```python
from build123d import *

# Parameters (mm, degrees)
EXTRUDE_1_DEPTH      = 3.7
EXTRUDE_1_DEPTH_BACK = 3.7
SKETCH_3_R           = 2.5
CUT_EXTRUDE_1_DEPTH  = 5
SKETCH_4_R           = 1.25
EXTRUDE_2_DEPTH      = 7
FILLET_1_R           = 1
FILLET_2_R           = 0.2


with BuildPart() as part:
    # 草图2 → 凸台-拉伸1 (new, two sides: drawn at the far end of the back side and taken through both)
    with BuildSketch(Plane(origin=(0, 0, 0), x_dir=(1, 0, 0), z_dir=(0, 1, 0)).offset(-EXTRUDE_1_DEPTH_BACK)):
        Polygon((12, 4.5), (12, -4.5), (0, -4.5), (-9, -4), (-13, -4), (-13, 4), (-9, 4), (0, 4.5), align=None)
    extrude(amount=EXTRUDE_1_DEPTH + EXTRUDE_1_DEPTH_BACK)

    # 草图3 → 切除-拉伸1 (cut)
    with BuildSketch(Plane(origin=(12, 0, 0), x_dir=(0, 0, -1), z_dir=(1, 0, 0))):
        Circle(SKETCH_3_R)
    extrude(amount=-CUT_EXTRUDE_1_DEPTH, mode=Mode.SUBTRACT)

    # 草图4 → 凸台-拉伸2 (add)
    with BuildSketch(Plane(origin=(7, 0, 0), x_dir=(0, 0, -1), z_dir=(1, 0, 0))):
        with Locations(Location((0, 0, 0), (0, 0, 180))):
            Circle(SKETCH_4_R)
    extrude(amount=EXTRUDE_2_DEPTH)

    # 圆角1
    fillet_1_edges = [part.edges().sort_by_distance(p)[0] for p in [
        (12, 0, -4.5),
        (12, 0, 4.5),
    ]]
    fillet(fillet_1_edges, radius=FILLET_1_R)

    # 圆角2
    fillet_2_edges = [part.edges().sort_by_distance(p)[0] for p in [
        (14, 0, -1.25),
    ]]
    fillet(fillet_2_edges, radius=FILLET_2_R)

    # 草图5 → 旋转1 (revolve)
    with BuildSketch(Plane(origin=(0, 0, 0), x_dir=(1, 0, 0), z_dir=(0, 1, 0))):
        Polygon((-13, 2.9), (-43, 2), (-43, 0), (-13, 0), align=None)
    revolve(axis=Axis((5.484305881, 0, 0), (-1, 0, 0)))


solid = part.part
```
For this review, take the finished solid that the model builds, in its own axes (mm). A direction names the side the tool comes from. Coordinates: 2 decimals unless noted, no trailing zeros. Write each loop counter-clockwise with the first axis right and the second up, starting at its lowest first coordinate (ties: lowest second). Pieces come first, ordered by that corner, then holes. Notation, with made-up numbers: (-31.75, 77.5) - (15.25, 77.5) arc R35 cw to (15.25, 111.5) - close; hole circle Ø6 at (67, -22.75). An arc over 180 degrees is marked (long way). Answer in a Markdown table with one row per item. Add a question column.
Q1. We need section A-A, the plane y = 0. State the section outline as (x, z) points.
Q2. Tool access review of faces 1 (the conical face through (-28.21, 2.386, 0.53)), 2 (the flat face through (7, -1, 1)), 3 (the flat face through (-11, 0, -4)), 4 (the flat face through (-11, 0, 4)): name each direction out of +Z, -Z, +X, -X, +Y, -Y from which nothing blocks a thin tool from reaching the whole face with its end or side.
Q3. For P1, Ø1.5, axis at y = -0.5, z = -1, coming from the +X side; P2, Ø2, axis at x = -11.5, y = 1, coming from the +Z side; P3, Ø1.2, axis at x = -11, y = 0.5, coming from the -Z side, all flat-tipped, find the tip position at first contact; note any pin that passes through.
Q4. We need section D-D, the plane x = -19.5. State the section outline as (y, z) points (3 decimals).
Q5. For probe 1 along Y at (x, z) = (9.4, 0); probe 2 along X at (y, z) = (3, 2); probe 3 along Z at (x, y) = (8, 2), list the stretches that pass through material, from the lowest coordinate up.
Q6. We need section B-B, the plane z = 0. State the section outline as (x, y) points, and give its area (3 significant figures).
Q7. We need section C-C, the plane x = -38. State the section outline as (y, z) points, and give its area (3 significant figures).
Q8. Draft analysis for pull direction Z (two halves, no side actions). For faces 5 (the cylindrical face through (10.35, -0.05, -1.25)), 6 (the flat face through (-4.563, -0.052, -4.246)), 7 (the flat face through (12, -3, 0)), state which applies: +Z half, -Z half, draft (parallel to the pull), parting line (faces both ways), or undercut.
Answer list:
| question | item | result |
|---|---|---|
| 1 | outline | (-43, -2) - (-13, -2.9) - (-13, -4) - (-9, -4) - (0, -4.5) - (11, -4.5) arc R1 ccw to (12, -3.5) - (12, -2.5) - (7, -2.5) - (7, -1.25) - (13.8, -1.25) arc R0.2 ccw to (14, -1.05) - (14, 1.05) arc R0.2 ccw to (13.8, 1.25) - (7, 1.25) - (7, 2.5) - (12, 2.5) - (12, 3.5) arc R1 ccw to (11, 4.5) - (0, 4.5) - (-9, 4) - (-13, 4) - (-13, 2.9) - (-43, 2) - close |
| 2 | face 1 | -X |
| 2 | face 2 | +X |
| 2 | face 3 | -Z, -X, +Y, -Y |
| 2 | face 4 | +Z, -X, +Y, -Y |
| 3 | P1 | stops at x = 14 |
| 3 | P2 | stops at z = 4 |
| 3 | P3 | stops at z = -4 |
| 4 | outline | circle Ø5.41 at (0, 0) |
| 5 | probe 1 | y = -3.7 to -2.5, -1.25 to 1.25, 2.5 to 3.7 |
| 5 | probe 2 | x = -13 to 12 |
| 5 | probe 3 | z = -4.5 to -1.5, 1.5 to 4.5 |
| 6 | outline | (-43, -2) - (-13, -2.9) - (-13, -3.7) - (12, -3.7) - (12, -2.5) - (7, -2.5) - (7, -1.25) - (13.8, -1.25) arc R0.2 ccw to (14, -1.05) - (14, 1.05) arc R0.2 ccw to (13.8, 1.25) - (7, 1.25) - (7, 2.5) - (12, 2.5) - (12, 3.7) - (-13, 3.7) - (-13, 2.9) - (-43, 2) - close |
| 6 | area | 324 mm2 |
| 7 | outline | circle Ø4.3 at (0, 0) |
| 7 | area | 14.5 mm2 |
| 8 | face 5 | undercut |
| 8 | face 6 | -Z half |
| 8 | face 7 | draft |
